from build123d import *

# Parameters (mm, degrees)
CROQUIS1_W              = 60
CROQUIS1_H              = 60
CROQUIS1_W_2            = 56
CROQUIS1_H_2            = 56
SALIENTE_EXTRUIR1_DEPTH = 221.22
CROQUIS3_W              = 60
CROQUIS3_H              = 60
CROQUIS3_W_2            = 56
CROQUIS3_H_2            = 56
SALIENTE_EXTRUIR2_DEPTH = 424.26
CORTAR_EXTRUIR1_DEPTH   = 61
CROQUIS14_W             = 60
CROQUIS14_H             = 60
CROQUIS14_W_2           = 56
CROQUIS14_H_2           = 56


with BuildPart() as part:
    # Croquis1 → Saliente-Extruir1 (new body)
    with BuildSketch(Plane(origin=(0, 0, 0), x_dir=(1, 0, 0), z_dir=(0, 1, 0))):
        Rectangle(CROQUIS1_W, CROQUIS1_H)
        Rectangle(CROQUIS1_W_2, CROQUIS1_H_2, mode=Mode.SUBTRACT)
    extrude(amount=SALIENTE_EXTRUIR1_DEPTH)



with BuildPart() as body_2:
    # Croquis3 → Saliente-Extruir2 (new body)
    with BuildSketch(Plane(origin=(15, -15, 0), x_dir=(0, 0, -1), z_dir=(0.707106781, -0.707106781, 0))):
        with Locations((0, -8.786796564)):
            Rectangle(CROQUIS3_W, CROQUIS3_H)
        with Locations((0, -8.786796564)):
            Rectangle(CROQUIS3_W_2, CROQUIS3_H_2, mode=Mode.SUBTRACT)
    extrude(amount=SALIENTE_EXTRUIR2_DEPTH)

    # Croquis10 → Cortar-Extruir1 (cut, through all)
    with BuildSketch(Plane.XY.offset(30)):
        Polygon((287.570716115, -342.423529857), (329.997122986, -299.997122986), (245.144309244, -299.997122986), align=None)
    extrude(amount=-CORTAR_EXTRUIR1_DEPTH, mode=Mode.SUBTRACT)


with BuildPart() as part_1:
    add(part.part)

    add(body_2.part)  # Barrer2 merges body 2
    # Barrer2: sweep along a path in Croquis13
    with BuildLine(Plane.XY.offset(30)) as barrer2_path:
        Line((-12.426406871, -42.426406871), (-30, 0))
    # Croquis14 → Barrer2 (sweep)
    with BuildSketch(Plane(origin=(15, -15, 0), x_dir=(0, 0, 1), z_dir=(-0.707106781, 0.707106781, 0))):
        with Locations((0, -8.786796564)):
            Rectangle(CROQUIS14_W, CROQUIS14_H)
        with Locations((0, -8.786796564)):
            Rectangle(CROQUIS14_W_2, CROQUIS14_H_2, mode=Mode.SUBTRACT)
    sweep(path=barrer2_path.line)


solid = part_1.part
Work out the finished part from the listing and answer in its coordinate system (mm). A direction names the side the tool comes from. Give positions to 0.01 mm unless a question says otherwise; leave off trailing zeros. Loops run counter-clockwise (first coordinate to the right, second up) from the corner with the lowest first, then second, coordinate; pieces in that order, holes last. Notation, with made-up numbers: (-19, 10.5) -> (11, 10.5) arc R13 cw to (11, 35.5) -> close; hole circle Ø1 at (88, 12). An arc over 180 degrees is marked (long way). Use a Markdown table: item, result. Add a question column.
1) Each of these flat-tipped pins is pushed along its axis until it touches: P1, Ø17, axis at y = 163.5, z = -12.5, coming from the +X side; P2, Ø4, axis at y = -70, z = -15, coming from the -X side; P3, Ø4, axis at y = -169.5, z = -12.5, coming from the +X side. Where does it stop, or does it pass through?
2) The part is cut by section C-C, the plane x = 146.5. Determine the outline of the cut face in (y, z), plus the area to 3 significant figures.
3) Consider line 1 along X through (y, z) = (177, 8); line 2 along X through (y, z) = (-229, 10). Determine where each line is inside the solid, lowest interval first.
4) For a pull along Z with two mould halves and no side action, classify faces 5 (the flat face through (114.56, -169.41, 0.42)), 6 (the flat face through (20.1, 23.9, 0.4)), 7 (the flat face through (92, -63, 30)) as +Z half, -Z half, draft (parallel to the pull), parting line (faces both ways), or undercut.
5) Which of the six approach directions +Z, -Z, +X, -X, +Y, -Y give full straight-line access (tool end or side, diameter ignored) to faces 1 (the flat face through (-19.625, -20.219, 0.392)), 2 (the flat face through (116.667, -168.692, 0.392)), 3 (the flat face through (291, -299.997, -29)), 4 (the flat face through (30, 109, 0))?
6) The part is cut by section B-B, the plane y = 110. Determine the outline of the cut face in (x, z).
7) The part is cut by section A-A, the plane z = 17. Determine the outline of the cut face in (x, y), plus the area to 3 significant figures.
8) The part is cut by section D-D, the plane y = 21. Determine the outline of the cut face in (x, z).
Reported:
| question | item | result |
|---|---|---|
| 1 | P1 | stops at x = 30 |
| 1 | P2 | stops at x = 13.15 |
| 1 | P3 | stops at x = 201.5 |
| 2 | outline | (-201.35, -30) -> (-116.5, -30) -> (-116.5, 30) -> (-201.35, 30) -> close; hole (-198.52, -28) -> (-119.33, -28) -> (-119.33, 28) -> (-198.52, 28) -> close |
| 2 | area | 656 mm^2 |
| 3 | line 1 | x = -30 to -28, 28 to 30 |
| 3 | line 2 | x = 174.15 to 176.98, 256.17 to 259 |
| 4 | face 5 | draft |
| 4 | face 6 | undercut |
| 4 | face 7 | +Z half |
| 5 | face 1 | +Y |
| 5 | face 2 | none |
| 5 | face 3 | +Z, -Z, +X, -X, -Y |
| 5 | face 4 | +Z, -Z, +X, +Y |
| 6 | outline | (-30, -30) -> (30, -30) -> (30, 30) -> (-30, 30) -> close; hole (-28, -28) -> (28, -28) -> (28, 28) -> (-28, 28) -> close |
| 7 | outline | (-30, 0) -> (-12.43, -42.43) -> (245.14, -300) -> (247.97, -300) -> (-11.01, -41.01) -> (-28, 0) -> (-28, 221.22) -> (-30, 221.22) -> close; (11.01, 41.01) -> (28.59, -1.41) -> (327.17, -300) -> (330, -300) -> (30, 0) -> (30, 221.22) -> (28, 221.22) -> (28, 4.83) -> (12.43, 42.43) -> close |
| 7 | area | 2,630 mm^2 |
| 8 | outline | (-30, -30) -> (30, -30) -> (30, 30) -> (-30, 30) -> close; hole (-28, -28) -> (19.3, -28) -> (19.3, 28) -> (-28, 28) -> close; hole (21.3, -28) -> (28, -28) -> (28, 28) -> (21.3, 28) -> close |
